Geometry check sheet. Reference: the model listing, model coordinates, mm. A direction names the side the tool comes from. Round coordinates to 2 decimals unless told otherwise and drop trailing zeros. Loops run counter-clockwise (first coordinate to the right, second up) from the corner with the lowest first, then second, coordinate; pieces in that order, holes last. Notation, with made-up numbers: (-8.5, 74.5) - (34.5, 74.5) arc R22 ccw to (34.5, 103.5) - close; hole circle Ø4 at (37.25, 51). An arc over 180 degrees is marked (long way). Answer as CSV lines item,"result". Start each with the question number.
1) Depth check by flat-ended pin: P1, Ø5, axis at x = -3.5, y = 11.5, coming from the +Z side; P2, Ø2, axis at x = 15, z = 0, coming from the +Y side. Enter the tip coordinate at first touch or a pass-through.
2) Draft check along Y on faces 4 (the cylindrical face through (15.75, -10.44, 0.05)), 5 (the conical face through (15.2, 9.88, 0.08)), 6 (the cylindrical face through (-18.52, -7.88, 0.27)). Enter one of: released by +Y, released by -Y, zero draft, split by the parting line, or undercut.
3) Cross-section at D-D on y = -0.25. Record the boundary of the cut face in (x, z).
4) Access from +Z, -Z, +X, -X, +Y, -Y to the whole of each face (thin tool, end or side, straight path). Record for faces 1 (the flat face through (12.2, 7, -1)), 2 (the cylindrical face through (18.52, 8.22, 0.27)), 3 (the cylindrical face through (-13.25, -10.44, 0.05)).
5) Cross-section at A-A on x = -5. Record the boundary of the cut face in (y, z), and give its area (3 significant figures).
6) Cross-section at B-B on z = 3. Record the boundary of the cut face in (x, y).
7) Cross-section at C-C on x = 11.2. Record the boundary of the cut face in (y, z).
8) Thickness scan on line 1 along Y through (x, z) = (3, 0); line 2 along Y through (x, z) = (17.65, 0); line 3 along X through (y, z) = (-11.25, 0). Record the ranges inside material, lowest first.
from build123d import *

# Parameters (mm, degrees)
SKETCH1_W                   = 40
SKETCH1_H                   = 30
BOSS_EXTRUDE1_DEPTH         = 4
CUT_EXTRUDE1_DEPTH          = 2
CUT_EXTRUDE2_DEPTH          = 26.709920264
M3_TAPPED_HOLE1_D           = 2.5
M3_TAPPED_HOLE1_DEPTH       = 9
M3_TAPPED_HOLE1_TIP         = 0.751075774
M3_TAPPED_HOLE2_AT_2_COUNT  = 2
M3_TAPPED_HOLE2_AT_2_PITCH  = 16.1
TAP_DRILL_FOR_M3_TAP1_D     = 2.5
TAP_DRILL_FOR_M3_TAP1_DEPTH = 4.5
TAP_DRILL_FOR_M3_TAP1_TIP   = 0.751075774


with BuildPart() as part:
    # Sketch1 → Boss-Extrude1 (new, symmetric)
    with BuildSketch(Plane.XY):
        Rectangle(SKETCH1_W, SKETCH1_H)
    extrude(amount=BOSS_EXTRUDE1_DEPTH, both=True)

    # Sketch2 → Cut-Extrude1 (cut)
    with BuildSketch(Plane.XY.offset(4)):
        with BuildLine():
            Line((-15.85, 21.25), (15.85, 21.25))
            ThreePointArc((15.85, 21.25), (16.910660172, 20.810660172), (17.35, 19.75))
            Line((17.35, 19.75), (17.35, -13.2))
            Line((17.35, -13.2), (17.35, -15))
            Line((17.35, -15), (-17.35, -15))
            Line((-17.35, -15), (-17.35, -13.2))
            Line((-17.35, -13.2), (-17.35, 19.75))
            ThreePointArc((-17.35, 19.75), (-16.910660172, 20.810660172), (-15.85, 21.25))
        make_face()
    extrude(amount=-CUT_EXTRUDE1_DEPTH, mode=Mode.SUBTRACT)

    # Sketch3 → Cut-Extrude2 (cut, through all)
    with BuildSketch(Plane.XY.offset(2)):
        with BuildLine():
            Line((12.2, 9.25), (12.2, 4.75))
            ThreePointArc((12.2, 4.75), (11.2, 3.75), (10.2, 4.75))
            Line((10.2, 4.75), (-10.2, 4.75))
            ThreePointArc((-10.2, 4.75), (-11.2, 3.75), (-12.2, 4.75))
            Line((-12.2, 4.75), (-12.2, 9.25))
            ThreePointArc((-12.2, 9.25), (-11.2, 10.25), (-10.2, 9.25))
            Line((-10.2, 9.25), (10.2, 9.25))
            ThreePointArc((10.2, 9.25), (11.2, 10.25), (12.2, 9.25))
        make_face()
        with BuildLine():
            Line((-10.2, -6.85), (10.2, -6.85))
            ThreePointArc((10.2, -6.85), (11.2, -5.85), (12.2, -6.85))
            Line((12.2, -6.85), (12.2, -11.35))
            ThreePointArc((12.2, -11.35), (11.2, -12.35), (10.2, -11.35))
            Line((10.2, -11.35), (-10.2, -11.35))
            ThreePointArc((-10.2, -11.35), (-11.2, -12.35), (-12.2, -11.35))
            Line((-12.2, -11.35), (-12.2, -6.85))
            ThreePointArc((-12.2, -6.85), (-11.2, -5.85), (-10.2, -6.85))
        make_face()
    extrude(amount=-CUT_EXTRUDE2_DEPTH, mode=Mode.SUBTRACT)

    # M3 Tapped Hole1
    with Locations(Plane(origin=(-0.662160093, -15, 0.523062075), x_dir=(1, 0, 0), z_dir=(0, -1, 0))):
        with Locations((15.162160093, -0.523062075), (-13.837839907, -0.523062075)):
            Hole(M3_TAPPED_HOLE1_D / 2, depth=M3_TAPPED_HOLE1_DEPTH)
            with Locations((0, 0, -(M3_TAPPED_HOLE1_DEPTH + M3_TAPPED_HOLE1_TIP / 2))):  # 118° drill point
                Cone(0, M3_TAPPED_HOLE1_D / 2, M3_TAPPED_HOLE1_TIP, mode=Mode.SUBTRACT)

    # Sketch16 → M3 Tapped Hole2 (revolve, cut)
    with BuildSketch(Plane(origin=(20, 7, 0), x_dir=(0, 0, -1), z_dir=(0, 1, 0))):
        Polygon((0, 0), (0, 3.751075774), (1.25, 3), (1.25, 0), align=None)
    m3_tapped_hole2 = revolve(axis=Axis((26.35, 7, 0), (-1, 0, 0)), mode=Mode.SUBTRACT)

    # M3 Tapped Hole2 at 2: M3 Tapped Hole2 ×2
    with Locations(*[(0, -i * M3_TAPPED_HOLE2_AT_2_PITCH, 0) for i in range(1, M3_TAPPED_HOLE2_AT_2_COUNT)]):
        add(m3_tapped_hole2, mode=Mode.SUBTRACT)

    # Mirror1: M3 Tapped Hole2 across plane
    add(m3_tapped_hole2.mirror(Plane(origin=(0, 0, 0), x_dir=(0, 0, 1), z_dir=(1, 0, 0))), mode=Mode.SUBTRACT)

    # Mirror1 copy 1 sketch → Mirror1 copy 1 (revolve, cut)
    with BuildSketch(Plane(origin=(-20, -9.1, 0), x_dir=(0, 0, -1), z_dir=(0, 1, 0))):
        Polygon((0, 0), (0, -3.751075774), (1.25, -3), (1.25, 0), align=None)
    revolve(axis=Axis((-26.35, -9.1, 0), (-1, 0, 0)), mode=Mode.SUBTRACT)

    # Tap Drill for M3 Tap1
    with Locations(Plane(origin=(0, 15, 0), x_dir=(1, 0, 0), z_dir=(0, 1, 0))):
        with Locations((-15, 0), (15, 0)):
            Hole(TAP_DRILL_FOR_M3_TAP1_D / 2, depth=TAP_DRILL_FOR_M3_TAP1_DEPTH)
            with Locations((0, 0, -(TAP_DRILL_FOR_M3_TAP1_DEPTH + TAP_DRILL_FOR_M3_TAP1_TIP / 2))):  # 118° drill point
                Cone(0, TAP_DRILL_FOR_M3_TAP1_D / 2, TAP_DRILL_FOR_M3_TAP1_TIP, mode=Mode.SUBTRACT)


solid = part.part
Answer block:
1,P1,"stops at z = 2"
1,P2,"stops at y = 10.35"
2,face 4,"zero draft"
2,face 5,"released by +Y"
2,face 6,"undercut"
3,outline,"(-20, -4) - (20, -4) - (20, 4) - (17.35, 4) - (17.35, 2) - (-17.35, 2) - (-17.35, 4) - (-20, 4) - close"
4,face 1,"+Z, -Z"
4,face 2,"+X"
4,face 3,"-Y"
5,outline,"(-15, -4) - (-11.35, -4) - (-11.35, 2) - (-15, 2) - close; (-6.85, -4) - (4.75, -4) - (4.75, 2) - (-6.85, 2) - close; (9.25, -4) - (15, -4) - (15, 2) - (9.25, 2) - close"
5,area,"126 mm^2"
6,outline,"(-20, -15) - (-17.35, -15) - (-17.35, 15) - (-20, 15) - close; (17.35, -15) - (20, -15) - (20, 15) - (17.35, 15) - close"
7,outline,"(-15, -4) - (-12.35, -4) - (-12.35, 2) - (-15, 2) - close; (-5.85, -4) - (3.75, -4) - (3.75, 2) - (-5.85, 2) - close; (10.25, -4) - (15, -4) - (15, 2) - (10.25, 2) - close"
8,line 1,"y = -15 to -11.35, -6.85 to 4.75, 9.25 to 15"
8,line 2,"y = -15 to -10.35, -7.85 to 5.75, 8.25 to 15"
8,line 3,"x = -20 to -15.75, -13.25 to -12.2, 12.2 to 13.25, 15.75 to 20"
